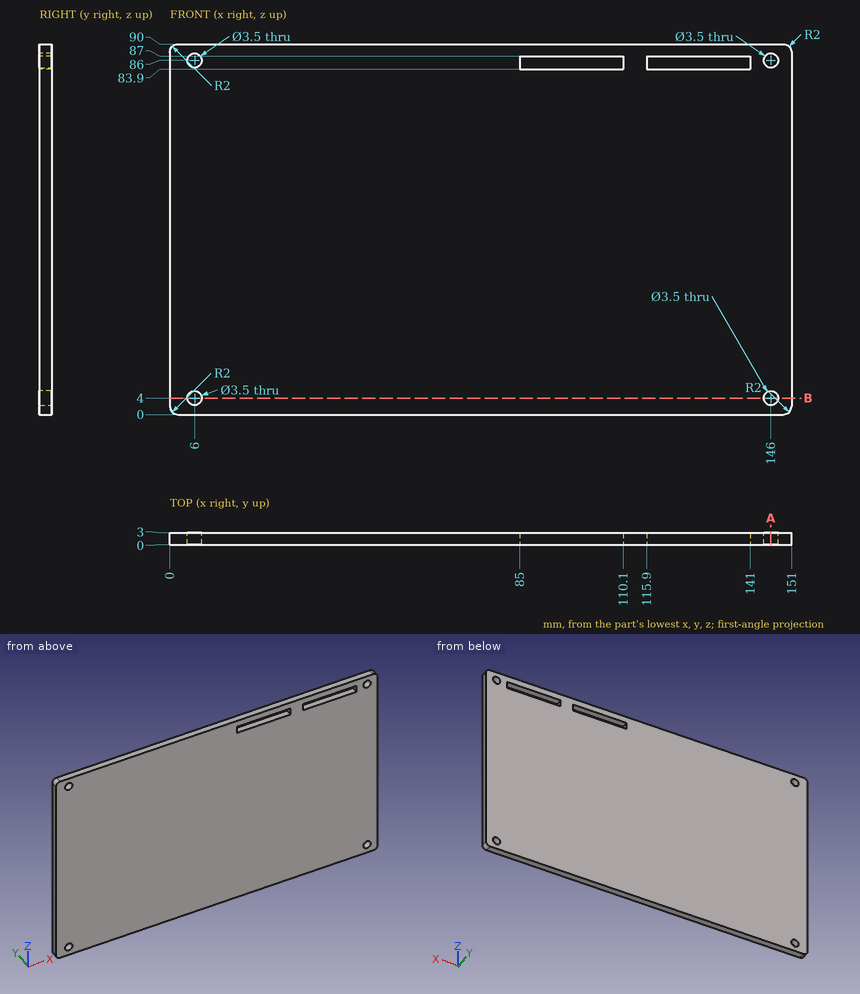
Source: three-view drawing plus pictorial views. Frame: mm from the lowest corner of the part. Round coordinates to 2 decimals unless told otherwise and drop trailing zeros. Order: outer loops, then holes, each group sorted by start corner. A loop starts at its lowest first (then second) coordinate and runs counter-clockwise, first axis right, second up. Notation, with made-up numbers: (-28.75, 47.5) - (14.25, 47.5) arc R10 cw to (14.25, 55.5) - close; hole circle Ø9 at (74, -30). An arc over 180 degrees is marked (long way). Answer in a Markdown table with one row per item.
Item 1: Section query A-A (x = 146). Return the cut outline in (y, z).
Model answer:
| item | result |
|---|---|
| outline | (0, 0) - (3, 0) - (3, 2.25) - (0, 2.25) - close; (0, 5.75) - (3, 5.75) - (3, 84.25) - (0, 84.25) - close; (0, 87.75) - (3, 87.75) - (3, 90) - (0, 90) - close |
Item 2: Section query B-B (z = 4). Return the cut outline in (x, y), then the cut area to 3 significant figures.
Model answer:
| item | result |
|---|---|
| outline | (0, 0) - (4.25, 0) - (4.25, 3) - (0, 3) - close; (7.75, 0) - (144.25, 0) - (144.25, 3) - (7.75, 3) - close; (147.75, 0) - (151, 0) - (151, 3) - (147.75, 3) - close |
| area | 432 mm² |
Item 3: Line query: line 1 (Z direction, x = 146, y = 2.1); line 2 (X direction, y = 2.25, z = 4); line 3 (X direction, y = 1.3, z = 86). Output: solid intervals per line, ascending.
Model answer:
| item | result |
|---|---|
| line 1 | z = 0 to 2.25, 5.75 to 84.25, 87.75 to 90 |
| line 2 | x = 0 to 4.25, 7.75 to 144.25, 147.75 to 151 |
| line 3 | x = 0 to 4.25, 7.75 to 85, 110.1 to 115.9, 141 to 144.25, 147.75 to 151 |
